Geometry: final body of the model. Coordinates: model frame, mm. Round coordinates to 2 decimals unless told otherwise and drop trailing zeros. One line per item, written item: value. Start each with the question number.
from build123d import *

# Parameters (mm, degrees)
SKETCH1_W           = 12
SKETCH1_H           = 10.5
BOSS_EXTRUDE1_DEPTH = 250
SKETCH2_R           = 3
CUT_EXTRUDE1_DEPTH  = 3.5
SKETCH3_R           = 1.75
CUT_EXTRUDE2_DEPTH  = 8
LPATTERN1_COUNT     = 12
LPATTERN1_PITCH     = 25


with BuildPart() as part:
    # Sketch1 → Boss-Extrude1 (new body)
    with BuildSketch(Plane.XY):
        with Locations((6, 5.25)):
            Rectangle(SKETCH1_W, SKETCH1_H)
    extrude(amount=BOSS_EXTRUDE1_DEPTH)

    # Sketch2 → Cut-Extrude1 (cut)
    with BuildSketch(Plane(origin=(0, 10.5, 0), x_dir=(1, 0, 0), z_dir=(0, 1, 0))):
        with Locations((6, -242.5)):
            Circle(SKETCH2_R)
    cut_extrude1 = extrude(amount=-CUT_EXTRUDE1_DEPTH, mode=Mode.SUBTRACT)

    # Sketch3 → Cut-Extrude2 (cut, through all)
    with BuildSketch(Plane(origin=(0, 7, 0), x_dir=(1, 0, 0), z_dir=(0, 1, 0))):
        with Locations((6, -242.5)):
            Circle(SKETCH3_R)
    cut_extrude2 = extrude(amount=-CUT_EXTRUDE2_DEPTH, mode=Mode.SUBTRACT)

    # LPattern1: Cut-Extrude1, Cut-Extrude2 ×12
    with Locations(*[(0, 0, -i * LPATTERN1_PITCH) for i in range(1, LPATTERN1_COUNT)]):
        add(cut_extrude1, mode=Mode.SUBTRACT)
        add(cut_extrude2, mode=Mode.SUBTRACT)


solid = part.part
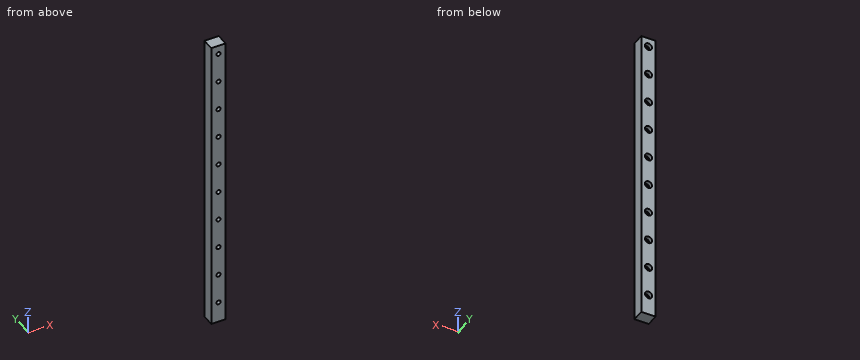
(1) Section query A-A (y = 5.25). Count the separate pieces of the cut face and the enclosed holes in it, and give its area (3 significant figures).
(2) Line query: probe 1 along X at (y, z) = (9.85, 17.5); probe 2 along Y at (x, z) = (8, 42); probe 3 along X at (y, z) = (2, 67.5). Output: solid intervals per line, ascending.
(3) Pin query (flat end, axial travel): pin 1 (2 mm diameter, centred on x = 6, z = 192.5, fed in from +Y); pin 2 (4.5 mm diameter, centred on x = 6, z = 142.5, fed in from +Y). Return the tip coordinate at first contact, or that it passes through.
Results list:
1. separate pieces: 1
1. enclosed holes: 10
1. area: 2,900 mm^2
2. probe 1: x = 0 to 3, 9 to 12
2. probe 2: y = 0 to 7
2. probe 3: x = 0 to 4.25, 7.75 to 12
3. pin 1: passes through
3. pin 2: stops at y = 7
